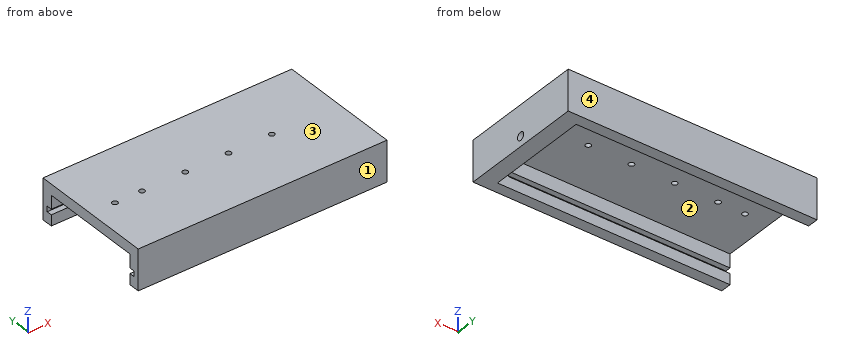
from build123d import *

# Parameters (mm, degrees)
F0_W     = 43
F0_H     = 19
F1_DEPTH = 2
F2_DEPTH = 5.5
F3_W     = 1
F3_H     = 1
F4_DEPTH = 41
F5_R     = 0.75
F6_DEPTH = 3
F7_R     = 0.5
F8_DEPTH = 2


with BuildPart() as f1:
    # F0 (on Top) → F1 (new body)
    with BuildSketch(Plane.XY):
        with Locations((17.1059944248, 8.7649840168)):
            Rectangle(F0_W, F0_H)
        Polygon((-4.3940055752, -0.7350159832), (-4.3940055752, -2.7350159832), (41.6059944248, -2.7350159832), (41.6059944248, 20.2649840168), (-4.3940055752, 20.2649840168), (-4.3940055752, 18.2649840168), (38.6059944248, 18.2649840168), (38.6059944248, -0.7350159832), align=None)
    extrude(amount=F1_DEPTH)

    # F0 (on Top) → F2 (join)
    with BuildSketch(Plane.XY):
        Polygon((-4.3940055752, -0.7350159832), (-4.3940055752, -2.7350159832), (41.6059944248, -2.7350159832), (41.6059944248, 20.2649840168), (-4.3940055752, 20.2649840168), (-4.3940055752, 18.2649840168), (38.6059944248, 18.2649840168), (38.6059944248, -0.7350159832), align=None)
    extrude(amount=-F2_DEPTH)

    # F3 (on face) → F4 (cut)
    with BuildSketch(Plane(origin=(-4.3940055752, 0, 0), x_dir=(0, -1, 0), z_dir=(-1, 0, 0))):
        with Locations((-18.7649840168, -3)):
            Rectangle(F3_W, F3_H)
        with Locations((1.2350159832, -3)):
            Rectangle(F3_W, F3_H)
    extrude(amount=-F4_DEPTH, mode=Mode.SUBTRACT)

    # F5 (on face) → F6 (cut, through all)
    with BuildSketch(Plane.YZ.offset(41.6059944248)):
        with Locations((8.7649840168, -3.65)):
            Circle(F5_R)
    extrude(amount=-F6_DEPTH, mode=Mode.SUBTRACT)

    # F7 (on face) → F8 (cut, through all)
    with BuildSketch(Plane.XY.offset(2)):
        with Locations((5.1059944248, 8.7649840168)):
            Circle(F7_R)
        with Locations((13.1059944248, 8.7649840168)):
            Circle(F7_R)
        with Locations((21.1059944248, 8.7649840168)):
            Circle(F7_R)
        with Locations((29.1059944248, 8.7649840168)):
            Circle(F7_R)
        with Locations((0.1059944248, 8.7649840168)):
            Circle(F7_R)
    extrude(amount=-F8_DEPTH, mode=Mode.SUBTRACT)


solid = f1.part
Build history of the part. All positions in model axes, mm. Face numbers are marked on the shaded views. Give positions to 0.01 mm unless a question says otherwise; leave off trailing zeros. Order: outer loops, then holes, each group sorted by start corner. A loop starts at its lowest first (then second) coordinate and runs counter-clockwise, first axis right, second up. Notation, with made-up numbers: M 24,59 L 76,59 A17 ccw 76,92 Z; hole C -37,4 d5. An arc over 180 degrees is marked long. Put each result on its own line as item: value.
Item 1: Two-plate mould, pull along Y, no slides. Class the marked faces 1, 2, 3 and 4: +Y half, -Y half, draft (parallel to the pull), parting line (faces both ways), or undercut.
From the geometry:
face 1: -Y half
face 2: undercut
face 3: draft
face 4: +Y half
Item 2: Flat gauge pins, fed straight in: pin 1 Ø1 at (y, z) = (14, -3.5) entering from -X; pin 2 Ø1.2 at (y, z) = (8.76, -3.65) entering from +X; pin 3 Ø0.5 at (y, z) = (-1, -3) entering from -X. Where does each tip first touch, or does it go through?
From the geometry:
pin 1: stops at x = 38.61
pin 2: passes through
pin 3: stops at x = 36.61
Item 3: Slice it at A-A, the plane y = 1.5. Write the cut outline in (x, z).
From the geometry:
outline: M -4.39,0 L 38.61,0 L 38.61,-5.5 L 41.61,-5.5 L 41.61,2 L -4.39,2 Z
Item 4: Probe line 1 (Y direction, x = 16, z = -3.75); line 2 (X direction, y = 1.5, z = -1); line 3 (Z direction, x = 6, y = -1). List the from-to ranges inside material, lowest first. Write a range as [from, to].
From the geometry:
line 1: y = [-2.74, -0.74], [18.26, 20.26]
line 2: x = [38.61, 41.61]
line 3: z = [-5.5, -3.5], [-2.5, 2]
Item 5: Slice it at B-B, the plane x = 31.5. Write the cut outline in (y, z).
From the geometry:
outline: M -2.74,-5.5 L -0.74,-5.5 L -0.74,-3.5 L -1.74,-3.5 L -1.74,-2.5 L -0.74,-2.5 L -0.74,0 L 18.26,0 L 18.26,-2.5 L 19.26,-2.5 L 19.26,-3.5 L 18.26,-3.5 L 18.26,-5.5 L 20.26,-5.5 L 20.26,2 L -2.74,2 Z
Item 6: Slice it at C-C, the plane z = -5. Write the cut outline in (x, y).
From the geometry:
outline: M -4.39,-2.74 L 41.61,-2.74 L 41.61,20.26 L -4.39,20.26 L -4.39,18.26 L 38.61,18.26 L 38.61,-0.74 L -4.39,-0.74 Z
